CAD build for the part. Positions are in the model's coordinates, mm. Face numbers are marked on the shaded views. A direction names the side the tool comes from. Give positions to 0.01 mm unless a question says otherwise; leave off trailing zeros. Write each loop counter-clockwise with the first axis right and the second up, starting at its lowest first coordinate (ties: lowest second). Pieces come first, ordered by that corner, then holes. Notation, with made-up numbers: (77, 64.25) - (135, 64.25) arc R31 cw to (135, 97.25) - close; hole circle Ø1 at (5.25, 14.25). An arc over 180 degrees is marked (long way). Answer as a JSON object with one key per item and string values.
Autodesk Inventor part; units mm, degrees
ref_plane "YZ Plane" through (0, 0, 0) normal (1, 0, 0) x (0, 1, 0)
ref_plane "XZ Plane" through (0, 0, 0) normal (0, 1, 0) x (-1, 0, 0)
ref_plane "XY Plane" through (0, 0, 0) normal (0, 0, 1) x (1, 0, 0)
sketch "スケッチ1" plane through (0, 0, 0) normal (0, 0, 1) x (1, 0, 0)
  circle A0 centre (0, 0) radius 7.5
  dimension "d0" = 15
extrude "押し出し1" add sketch "スケッチ1" along normal blind 1
sketch "スケッチ2" plane through (0, 0, 1) normal (0, 0, 1) x (1, 0, 0)
  circle A0 centre (0, 0) radius 5
  dimension "d3" = 10
extrude "押し出し2" add sketch "スケッチ2" along normal blind 2.8
sketch "スケッチ3" plane through (0, 0, 3.8) normal (0, 0, 1) x (1, 0, 0)
  circle A0 centre (0, 0) radius 5
  circle A1 centre (0, 0) radius 5
  circle A2 centre (0, 0) radius 4
  dimension "d6" = 8
extrude "押し出し3" cut sketch "スケッチ3" against normal through all contours A2
properties part number "oiles_bush8" material "ABS プラスチック"
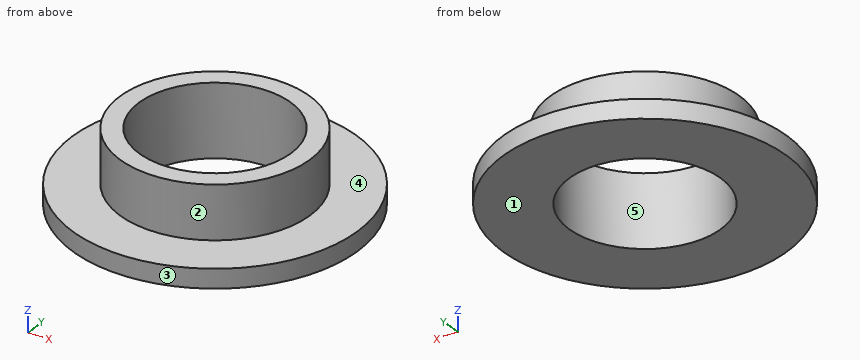
Item 1: Which spindle directions (+Z, -Z, +X, -X, +Y, -Y) get a long thin tool onto all of the face, cutting with end or side? Do the marked faces 1 and 2. Say none if no direction does.
Entries:
{"face 1": "-Z, +X, -X, +Y, -Y", "face 2": "+Z"}
Item 2: Flat gauge pins, fed straight in: P1, Ø6, axis at x = 6, y = 5.5, coming from the +Z side; P2, Ø9, axis at x = 0, y = 0, coming from the +Z side. Where does each tip first touch, or does it go through?
Entries:
{"P1": "z = 1", "P2": "z = 3.8"}
Item 3: Cut at D-D (y = 4.5). Give the cut face in (x, z), and give its area (3 significant figures).
Entries:
{"outline": "(-6, 0) - (6, 0) - (6, 1) - (2.18, 1) - (2.18, 3.8) - (-2.18, 3.8) - (-2.18, 1) - (-6, 1) - close", "area": "24.2 mm2"}
Item 4: Cut at A-A (y = 0). Give the cut face in (x, z), and give its area (3 significant figures).
Entries:
{"outline": "(-7.5, 0) - (-4, 0) - (-4, 3.8) - (-5, 3.8) - (-5, 1) - (-7.5, 1) - close; (4, 0) - (7.5, 0) - (7.5, 1) - (5, 1) - (5, 3.8) - (4, 3.8) - close", "area": "12.6 mm2"}
Item 5: Mould opens along X. For the marked faces 3, 4 and 5 say: +X half, -X half, draft (parallel to the pull), parting line (faces both ways), or undercut.
Entries:
{"face 3": "parting line", "face 4": "draft", "face 5": "undercut"}
Item 6: Cut at C-C (z = 2.4). Give the cut face in (x, y), and give its area (3 significant figures).
Entries:
{"outline": "circle Ø10 at (0, 0); hole circle Ø8 at (0, 0)", "area": "28.3 mm2"}
Item 7: Probe line 1 (Y direction, x = 0, z = 1.9); line 2 (Z direction, x = 1, y = 5.75); line 3 (X direction, y = -2.5, z = 1.2). List the from-to ranges inside material, lowest first. Write a range as from..to.
Entries:
{"line 1": "-5..-4, 4..5", "line 2": "0..1", "line 3": "-4.33..-3.12, 3.12..4.33"}
